Study the drawing (mm; zero at the part's minimum x, y, z) and answer. Coordinates: 2 decimals unless noted, no trailing zeros. Order: outer loops, then holes, each group sorted by start corner. A loop starts at its lowest first (then second) coordinate and runs counter-clockwise, first axis right, second up. Notation, with made-up numbers: (78.25, 18) -> (100.25, 18) arc R31 cw to (100.25, 42) -> close; hole circle Ø4 at (14.25, 87.5). An arc over 180 degrees is marked (long way). Put each result on its own line as item: value. Start each with the question number.
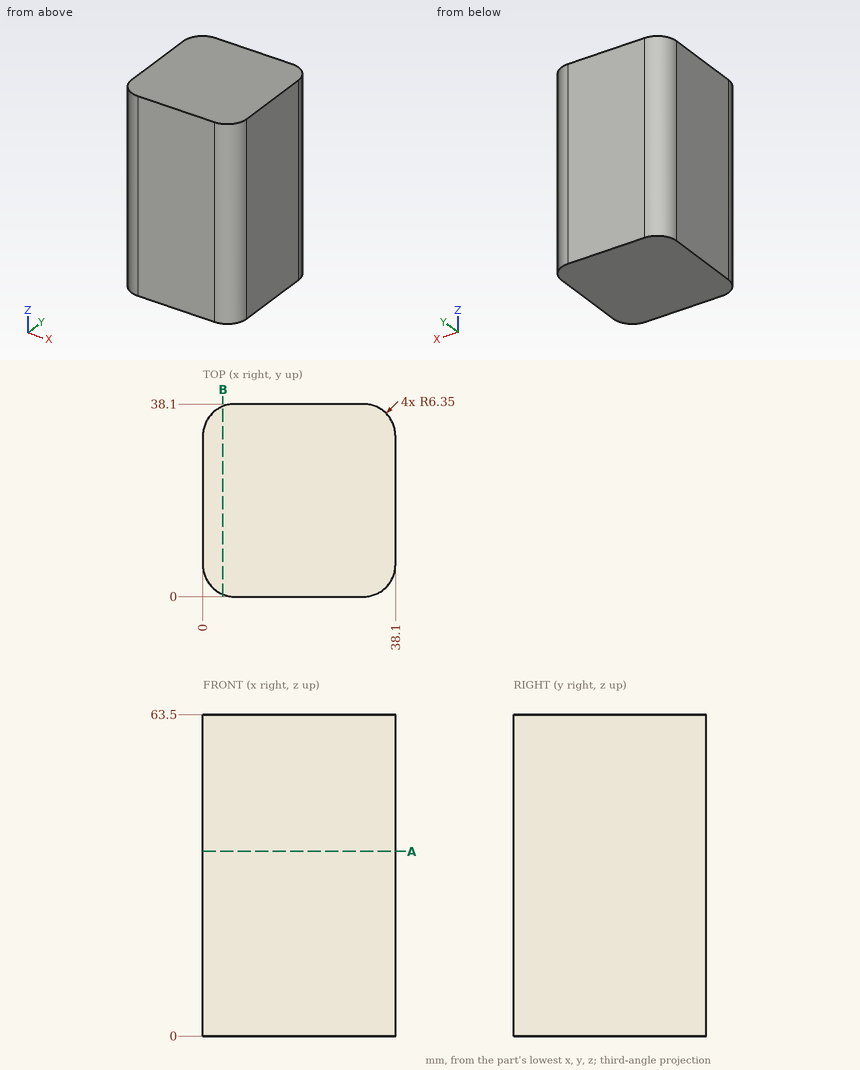
(1) The part is cut by section A-A on z = 36.5. Determine the outline of the cut face in (x, y).
(2) Find the intervals of material crossed by L1, parallel to Y at x = 36.5, z = 29; L2, parallel to Y at x = 3, z = 55; L3, parallel to X at y = 36, z = 24.5, in increasing order.
(3) The part is cut by section B-B on x = 4. Determine the outline of the cut face in (y, z), plus the area to 3 significant figures.
Worked out:
1. outline: (0, 6.35) arc R6.35 ccw to (6.35, 0) -> (31.75, 0) arc R6.35 ccw to (38.1, 6.35) -> (38.1, 31.75) arc R6.35 ccw to (31.75, 38.1) -> (6.35, 38.1) arc R6.35 ccw to (0, 31.75) -> close
2. L1: 2.14 to 35.96
2. L2: 0.96 to 37.14
2. L3: 1.63 to 36.47
3. outline: (0.45, 0) -> (37.65, 0) -> (37.65, 63.5) -> (0.45, 63.5) -> close
3. area: 2,360 mm2
